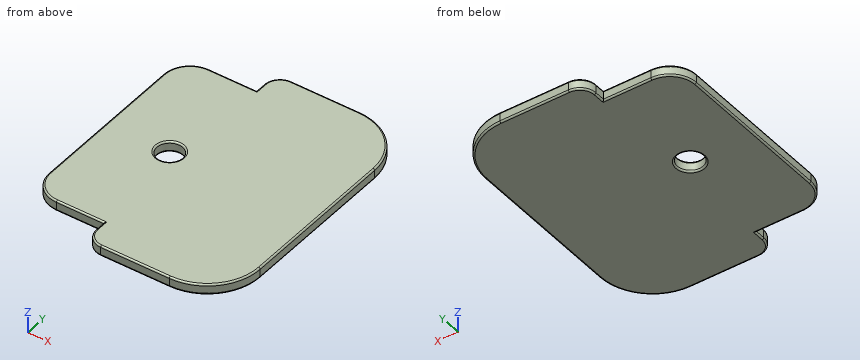
from build123d import *

# Parameters (mm, degrees)
F0_R     = 24.5
F1_DEPTH = 20
F2_R     = 3


with BuildPart() as f1:
    # F0 (on Top) → F1 (new body)
    with BuildSketch(Plane.XY):
        with BuildLine():
            Line((-30, -250), (100, -250))
            ThreePointArc((100, -250), (170.710678, -220.710678), (200, -150))
            Line((200, -150), (200, 150))
            ThreePointArc((200, 150), (170.710678, 220.710678), (100, 250))
            Line((100, 250), (-30, 250))
            ThreePointArc((-30, 250), (-51.213203, 241.213203), (-60, 220))
            Line((-60, 220), (-60, 200))
            Line((-60, 200), (-150, 200))
            ThreePointArc((-150, 200), (-185.355339, 185.355339), (-200, 150))
            Line((-200, 150), (-200, -150))
            ThreePointArc((-200, -150), (-185.355339, -185.355339), (-150, -200))
            Line((-150, -200), (-60, -200))
            Line((-60, -200), (-60, -220))
            ThreePointArc((-60, -220), (-51.213203, -241.213203), (-30, -250))
        make_face()
        with Locations((-80, 0)):
            Circle(F0_R, mode=Mode.SUBTRACT)
    extrude(amount=F1_DEPTH)

    # F2
    f2_edges = [f1.edges().sort_by_distance(p)[0] for p in [
        (-185.355339, -185.355339, 20),
        (-105, -200, 20),
        (-60, -210, 20),
        (-51.213203, -241.213203, 20),
        (35, -250, 20),
        (170.710678, -220.710678, 20),
        (200, 0, 20),
        (170.710678, 220.710678, 20),
        (35, 250, 20),
        (-51.213203, 241.213203, 20),
        (-60, 210, 20),
        (-105, 200, 20),
        (-185.355339, 185.355339, 20),
        (-200, 0, 20),
        (-104.5, 0, 20),
        (-185.355339, -185.355339, 0),
        (-105, -200, 0),
        (-60, -210, 0),
        (-51.213203, -241.213203, 0),
        (35, -250, 0),
        (170.710678, -220.710678, 0),
        (200, 0, 0),
        (170.710678, 220.710678, 0),
        (35, 250, 0),
        (-51.213203, 241.213203, 0),
        (-60, 210, 0),
        (-105, 200, 0),
        (-185.355339, 185.355339, 0),
        (-200, 0, 0),
        (-104.5, 0, 0),
    ]]
    fillet(f2_edges, radius=F2_R)


solid = f1.part
Check sheet for the modelled part. Datum: model origin and axes. Units: mm. Round coordinates to 2 decimals unless told otherwise and drop trailing zeros. Write each loop counter-clockwise with the first axis right and the second up, starting at its lowest first coordinate (ties: lowest second). Pieces come first, ordered by that corner, then holes. Notation, with made-up numbers: (46.5, 52.5) -> (92.5, 52.5) arc R7 ccw to (92.5, 59.5) -> close; hole circle Ø7 at (-25.5, 75). An arc over 180 degrees is marked (long way). Answer as CSV lines item,"result". Start each with the question number.
1) Section check D-D on x = -120. Enter the section's corners in (y, z), and give its area (3 significant figures).
2) Go/stop test with flat-tipped pins: P1, Ø4, axis at y = -209, z = 10.5, coming from the -X side; P2, Ø11, axis at x = -100, z = 10, coming from the +Y side; P3, Ø4, axis at x = 150, z = 8, coming from the +Y side. Record where each tip stops, or that it passes through.
3) Material ranges on line 1 (Y direction, x = -80, z = 6.5); line 2 (Y direction, x = -123.5, z = 3); line 3 (Y direction, x = 16, z = 17.25), recorded low to high. Write a range as from..to.
4) Section check C-C on y = 0. Enter the section's corners in (x, z), and give its area (3 significant figures).
5) Section check A-A on x = -80. Enter the section's corners in (y, z).
6) Section check B-B on z = 7.5. Enter the section's corners in (x, y).
Found:
1,outline,"(-200, 3) arc R3 ccw to (-197, 0) -> (197, 0) arc R3 ccw to (200, 3) -> (200, 17) arc R3 ccw to (197, 20) -> (-197, 20) arc R3 ccw to (-200, 17) -> close"
1,area,"7,990 mm^2"
2,P1,"stops at x = -60"
2,P2,"stops at y = 200"
2,P3,"stops at y = 237.73"
3,line 1,"y = -200..-24.5, 24.5..200"
3,line 2,"y = -200..200"
3,line 3,"y = -249.99..249.99"
4,outline,"(-200, 3) arc R3 ccw to (-197, 0) -> (-107.5, 0) arc R3 ccw to (-104.5, 3) -> (-104.5, 17) arc R3 ccw to (-107.5, 20) -> (-197, 20) arc R3 ccw to (-200, 17) -> close; (-55.5, 3) arc R3 ccw to (-52.5, 0) -> (197, 0) arc R3 ccw to (200, 3) -> (200, 17) arc R3 ccw to (197, 20) -> (-52.5, 20) arc R3 ccw to (-55.5, 17) -> close"
4,area,"7,000 mm^2"
5,outline,"(-200, 3) arc R3 ccw to (-197, 0) -> (-27.5, 0) arc R3 ccw to (-24.5, 3) -> (-24.5, 17) arc R3 ccw to (-27.5, 20) -> (-197, 20) arc R3 ccw to (-200, 17) -> close; (24.5, 3) arc R3 ccw to (27.5, 0) -> (197, 0) arc R3 ccw to (200, 3) -> (200, 17) arc R3 ccw to (197, 20) -> (27.5, 20) arc R3 ccw to (24.5, 17) -> close"
6,outline,"(-200, -150) arc R50 ccw to (-150, -200) -> (-60, -200) -> (-60, -220) arc R30 ccw to (-30, -250) -> (100, -250) arc R100 ccw to (200, -150) -> (200, 150) arc R100 ccw to (100, 250) -> (-30, 250) arc R30 ccw to (-60, 220) -> (-60, 200) -> (-150, 200) arc R50 ccw to (-200, 150) -> close; hole circle Ø49 at (-80, 0)"
